Design review of the part shown in the three views and the two pictorial views. Dimensions are in mm from the part's minimum x, y and z. Round coordinates to 2 decimals unless told otherwise and drop trailing zeros. Loops run counter-clockwise (first coordinate to the right, second up) from the corner with the lowest first, then second, coordinate; pieces in that order, holes last.
1. To check wall thickness, follow line 1 along Y through (x, z) = (8.25, 6) (3 decimals). State the ranges of the line that lie inside material, in increasing order.
2. Consider section A-A on x = 12.5. State the section outline as (y, z) points (3 decimals), then the cut area to 3 significant figures.
3. Consider section B-B on z = 4.5. State the section outline as (x, y) points (3 decimals).
4. Clearance check with flat-ended pins moving along their axes: pin 1 Ø1 at (x, z) = (8, 4) entering from +Y (3 decimals); pin 2 Ø0.9 at (y, z) = (0, 0.5) entering from +X (3 decimals). State where each tip first meets the part, or that it passes through.
5. Consider section C-C on x = 6. State the section outline as (y, z) points (3 decimals), then the cut area to 3 significant figures.
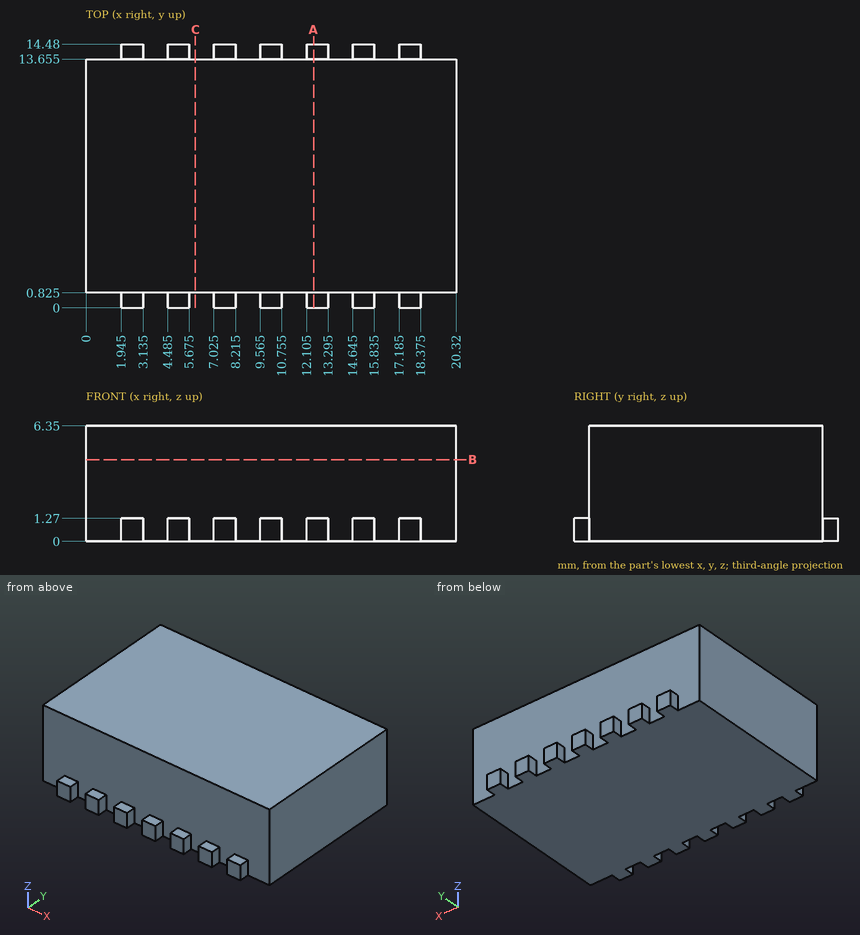
Resolved:
1. line 1: y = 0.825 to 13.655
2. outline: (0, 0) - (14.48, 0) - (14.48, 1.27) - (13.655, 1.27) - (13.655, 6.35) - (0.825, 6.35) - (0.825, 1.27) - (0, 1.27) - close
2. area: 83.6 mm2
3. outline: (0, 0.825) - (20.32, 0.825) - (20.32, 13.655) - (0, 13.655) - close
4. pin 1: stops at y = 13.655
4. pin 2: stops at x = 18.375
5. outline: (0.825, 0) - (13.655, 0) - (13.655, 6.35) - (0.825, 6.35) - close
5. area: 81.5 mm2
